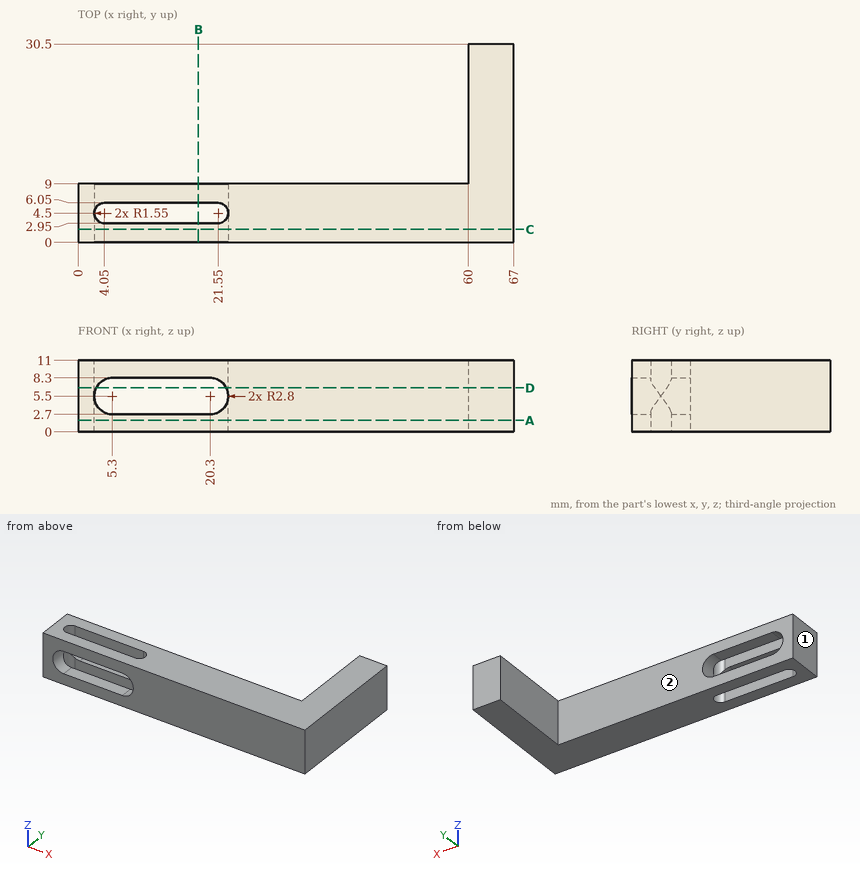
Check sheet for the drawn part. Datum: minimum x, y, z corner. Units: mm. A direction names the side the tool comes from. Coordinates: 2 decimals unless noted, no trailing zeros. Order: outer loops, then holes, each group sorted by start corner. A loop starts at its lowest first (then second) coordinate and runs counter-clockwise, first axis right, second up. Notation, with made-up numbers: M 77,39 L 87,39 A25 ccw 87,51 Z; hole C 58.25,-25.5 d4. An arc over 180 degrees is marked long. One line per question, with ' | ' between items. Start each with the question number.
Item 1: Sectioned sample at B-B on x = 18.5. Record the cut outline in (y, z), and give its area (3 significant figures).
Item 2: Sectioned sample at A-A on z = 1.75. Record the cut outline in (x, y).
Item 3: Access from +Z, -Z, +X, -X, +Y, -Y to the whole of each face (thin tool, end or side, straight path). Record for the marked faces 1 and 2.
Item 4: Sectioned sample at D-D on z = 6.75. Record the cut outline in (x, y), and give its area (3 significant figures).
Item 5: Sectioned sample at C-C on y = 2. Record the cut outline in (x, z).
Item 6: Material ranges on line 1 (Z direction, x = 9.5, y = 7.5); line 2 (Y direction, x = 19.5, z = 2.25); line 3 (X direction, y = 20, z = 5.25), recorded low to high.
Item 7: Gauge pin test, flat ends, axial feed: P1, Ø3.5, axis at y = 22.5, z = 7.5, coming from the -X side; P2, Ø3.5, axis at x = 14, z = 1, coming from the +Y side. Record the tip position at first contact, or that the pin passes through.
Answer below:
1) outline: M 0,0 L 2.95,0 L 2.95,2.7 L 0,2.7 Z; M 0,8.3 L 2.95,8.3 L 2.95,11 L 0,11 Z; M 6.05,0 L 9,0 L 9,2.7 L 6.05,2.7 Z; M 6.05,8.3 L 9,8.3 L 9,11 L 6.05,11 Z | area: 31.9 mm^2
2) outline: M 0,0 L 67,0 L 67,30.5 L 60,30.5 L 60,9 L 0,9 Z; hole M 4.05,2.95 L 21.55,2.95 A1.55 ccw 21.55,6.05 L 4.05,6.05 A1.55 ccw Z
3) face 1: +Z, -Z, -X, +Y, -Y | face 2: +Z, -Z, -X, +Y
4) outline: M 0,0 L 2.79,0 L 2.79,3.59 A1.55 cw 2.79,5.41 L 2.79,9 L 0,9 Z; M 22.81,0 L 67,0 L 67,30.5 L 60,30.5 L 60,9 L 22.81,9 L 22.81,5.41 A1.55 cw 22.81,3.59 Z | area: 573 mm^2
5) outline: M 0,0 L 67,0 L 67,11 L 0,11 Z; hole M 5.3,2.7 L 20.3,2.7 A2.8 ccw 20.3,8.3 L 5.3,8.3 A2.8 ccw Z
6) line 1: z = 0 to 2.7, 8.3 to 11 | line 2: y = 0 to 2.95, 6.05 to 9 | line 3: x = 60 to 67
7) P1: stops at x = 60 | P2: stops at y = 9
